Geometry: final body of the model. Coordinates: model frame, mm. Give positions to 0.01 mm unless a question says otherwise; leave off trailing zeros. Write each loop counter-clockwise with the first axis right and the second up, starting at its lowest first coordinate (ties: lowest second). Pieces come first, ordered by that corner, then holes. Notation, with made-up numbers: M 72.25,37.25 L 120.25,37.25 A12 ccw 120.25,51.25 Z; hole C -15.75,63 d7. An arc over 180 degrees is marked long. Use a Markdown table: item, result. Add a question column.
(1) Draft query along X for faces 1 (the cylindrical face through (-21, 11, -28)), 2 (the cylindrical face through (-86.5, 11.34, 44.99)), 3 (the flat face through (-42, 23, -1)). Return one class per face: released by +X, released by -X, zero draft, split by the parting line, or undercut.
(2) Cut plane C-C (y = 6.5). Output: boundary loops of the cut face in (x, z), plus the area to 3 significant figures.
(3) Material intervals for L1, parallel to X at y = 14.25, z = 0; L2, parallel to Z at x = 23, y = 3.5; L3, parallel to Z at x = 22, y = 2.25, sorted ascending.
(4) Pin query (flat end, axial travel): pin 1 Ø2.5 at (x, z) = (22.1, -38.27) entering from +Y; pin 2 Ø10 at (x, y) = (-8.5, 9.5) entering from +Z; pin 3 Ø4 at (x, y) = (-70, 8.5) entering from +Z. Return the tip coordinate at first contact, or that it passes through.
(5) Cut plane D-D (z = 66). Output: boundary loops of the cut face in (x, y).
(6) Cut plane B-B (z = -11). Output: boundary loops of the cut face in (x, y).
(7) Cut plane A-A (x = 0). Output: boundary loops of the cut face in (y, z).
```python
from build123d import *

# Parameters (mm, degrees)
SKETCH1_R             = 97.5
BOSS_EXTRUDE1_DEPTH   = 23
SKETCH2_R             = 35
CUT_EXTRUDE1_DEPTH    = 140.790915299
SKETCH3_R             = 1.668376245
CUT_EXTRUDE2_DEPTH    = 21.971332
CIRPATTERN1_START     = 1.028667902
CIRPATTERN1_OUTLINE_R = 1.668376245
CIRPATTERN1_DEPTH     = 21.971332098


# Read off the part's stored shape, not the designer's step: CirPattern1
with BuildPart() as part:
    # Sketch1 → Boss-Extrude1 (new body)
    with BuildSketch(Plane(origin=(0, 0, 0), x_dir=(1, 0, 0), z_dir=(0, 1, 0))):
        with Locations(Location((0, 0, 0), (0, 0, 270))):
            Circle(SKETCH1_R)
    extrude(amount=BOSS_EXTRUDE1_DEPTH)

    # Sketch2 → Cut-Extrude1 (cut, through all)
    with BuildSketch(Plane(origin=(0, 0, 0), x_dir=(1, 0, 0), z_dir=(0, 1, 0))):
        with Locations(Location((0, 0, 0), (0, 0, 270))):
            Circle(SKETCH2_R)
    extrude(amount=CUT_EXTRUDE1_DEPTH, mode=Mode.SUBTRACT)

    # Sketch3 → Cut-Extrude2 (cut)
    with BuildSketch(Plane(origin=(0, 23, 0), x_dir=(1, 0, 0), z_dir=(0, 1, 0))):
        with Locations(Location((-44.195851492, 0, 0), (0, 0, 270))):
            Circle(SKETCH3_R)
    extrude(amount=-CUT_EXTRUDE2_DEPTH, mode=Mode.SUBTRACT)

    # CirPattern1 outline → CirPattern1 (cut)
    with BuildSketch(Plane(origin=(0, 0, 0), x_dir=(1, 0, 0), z_dir=(0, 1, 0)).offset(CIRPATTERN1_START)):
        with Locations((22.097925746, 38.274730134)):
            Circle(CIRPATTERN1_OUTLINE_R)
        with Locations((22.097925746, -38.274730134)):
            Circle(CIRPATTERN1_OUTLINE_R)
    extrude(amount=CIRPATTERN1_DEPTH, mode=Mode.SUBTRACT)


solid = part.part
```
Answer list:
| question | item | result |
|---|---|---|
| 1 | face 1 | undercut |
| 1 | face 2 | split by the parting line |
| 1 | face 3 | zero draft |
| 2 | outline | C 0,0 d195; hole C -44.2,0 d3.34; hole C 0,0 d70; hole C 22.1,-38.27 d3.34; hole C 22.1,38.27 d3.34 |
| 2 | area | 26,000 mm² |
| 3 | L1 | -97.5 to -45.86, -42.53 to -35, 35 to 97.5 |
| 3 | L2 | -94.75 to -39.68, -36.87 to -26.38, 26.38 to 36.87, 39.68 to 94.75 |
| 3 | L3 | -94.99 to -39.94, -36.61 to -27.22, 27.22 to 36.61, 39.94 to 94.99 |
| 4 | pin 1 | y = 1.03 |
| 4 | pin 2 | z = 97.44 |
| 4 | pin 3 | z = 69.87 |
| 5 | outline | M -71.77,0 L 71.77,0 L 71.77,23 L -71.77,23 Z |
| 6 | outline | M -96.88,0 L -33.23,0 L -33.23,23 L -96.88,23 Z; M 33.23,0 L 96.88,0 L 96.88,23 L 33.23,23 Z |
| 7 | outline | M 0,-97.5 L 23,-97.5 L 23,-35 L 0,-35 Z; M 0,35 L 23,35 L 23,97.5 L 0,97.5 Z |
